The model under review builds one solid part; all positions refer to its coordinate system, in mm. A direction names the side the tool comes from. Coordinates: 2 decimals unless noted, no trailing zeros. Write each loop counter-clockwise with the first axis right and the second up, starting at its lowest first coordinate (ties: lowest second). Pieces come first, ordered by that corner, then holes. Notation, with made-up numbers: (74.5, 53) - (117.5, 53) arc R11 ccw to (117.5, 69) - close; hole circle Ø6 at (37.25, -14.75). An arc over 180 degrees is marked (long way). Put each result on its own line as item: value. Start each with the question number.
Item 1: Mouldability with a two-part tool opening along X and no side actions: class faces 1 (the face through (7, 0, 20)), 2 (the face through (-28, -21, 15)), 3 (the face through (18.34, 1.05, 17.46)) as pulls with the +X half, pulls with the -X half, needs draft (parallel to the pull), parting line crosses it, or undercut.
Item 2: Machinability: for faces 4 (the face through (-11.66, 1.05, 17.46)), 5 (the face through (8, 0, 12)), which of the approach directions +Z, -Z, +X, -X, +Y, -Y give a long, thin tool a straight path to every point of the face, cutting with its end or side? Answer none if there is none.
Item 3: Consider section B-B on z = 16.5. Give the boundary of the cut face in (x, y), then the cut area to 3 significant figures.
Item 4: Consider section A-A on x = 0. Give the boundary of the cut face in (y, z), then the cut area to 3 significant figures.
Item 5: To check wall thickness, follow L1, parallel to Y at x = 25, z = 15; L2, parallel to Y at x = 15, z = 18.8; L3, parallel to X at y = 14, z = 17.75. State the ranges of each line that lie inside material, in increasing order. Write a range as [from, to].
Item 6: For pin 1 (3 mm diameter, centred on x = 9, z = 16.5, fed in from -Y); pin 2 (8.5 mm diameter, centred on x = 15, y = 0, fed in from -Z); pin 3 (6 mm diameter, centred on x = -18, z = 16.5, fed in from -Y), all flat-tipped, find the tip position at first contact; note any pin that passes through.
```python
from build123d import *

# Parameters (mm, degrees)
CYLINDER001_R        = 3.5
CYLINDER001_DEPTH    = 10
CYLINDER002_R        = 7
CYLINDER002_DEPTH    = 5
CYLINDER003_R        = 3.5
CYLINDER003_DEPTH    = 10
CYLINDER004_R        = 7
CYLINDER004_DEPTH    = 5
CYLINDER005_R        = 2.6
CYLINDER005_DEPTH    = 10
CYLINDER006_R        = 2.6
CYLINDER006_DEPTH    = 10
CYLINDER_R           = 3
CYLINDER_DEPTH       = 10
CYLINDER001027_R     = 35
CYLINDER001027_DEPTH = 10
CHAMFER004_SIZE      = 1


with BuildPart() as cylinder001:
    # cylinder001 → cylinder001 (new body)
    with BuildSketch(Plane(origin=(15, 0, 0), x_dir=(1, 0, 0), z_dir=(0, 0, 1))):
        Circle(CYLINDER001_R)
    extrude(amount=CYLINDER001_DEPTH)


with BuildPart() as cylinder002:
    # cylinder002 → cylinder002 (new body)
    with BuildSketch(Plane(origin=(15, 0, 0), x_dir=(1, 0, 0), z_dir=(0, 0, 1))):
        Circle(CYLINDER002_R)
    extrude(amount=CYLINDER002_DEPTH)


with BuildPart() as cylinder003:
    # cylinder003 → cylinder003 (new body)
    with BuildSketch(Plane(origin=(-15, 0, 0), x_dir=(1, 0, 0), z_dir=(0, 0, 1))):
        Circle(CYLINDER003_R)
    extrude(amount=CYLINDER003_DEPTH)


with BuildPart() as cylinder004:
    # cylinder004 → cylinder004 (new body)
    with BuildSketch(Plane(origin=(-15, 0, 0), x_dir=(1, 0, 0), z_dir=(0, 0, 1))):
        Circle(CYLINDER004_R)
    extrude(amount=CYLINDER004_DEPTH)


with BuildPart() as cylinder005:
    # cylinder005 → cylinder005 (new body)
    with BuildSketch(Plane(origin=(-25, 0, 0), x_dir=(1, 0, 0), z_dir=(0, 0, 1))):
        Circle(CYLINDER005_R)
    extrude(amount=CYLINDER005_DEPTH)


with BuildPart() as cylinder006:
    # cylinder006 → cylinder006 (new body)
    with BuildSketch(Plane(origin=(25, 0, 0), x_dir=(1, 0, 0), z_dir=(0, 0, 1))):
        Circle(CYLINDER006_R)
    extrude(amount=CYLINDER006_DEPTH)


with BuildPart() as union:
    # cylinder → cylinder (new body)
    with BuildSketch(Plane.XY):
        Circle(CYLINDER_R)
    extrude(amount=CYLINDER_DEPTH)

    # union: union cylinder001, cylinder002, cylinder003, cylinder004, cylinder005, cylinder006
    add(cylinder001.part)
    add(cylinder002.part)
    add(cylinder003.part)
    add(cylinder004.part)
    add(cylinder005.part)
    add(cylinder006.part)


with BuildPart() as obj1:
    # Cylinder001027 → Cylinder001027 (new body)
    with BuildSketch(Plane.XY):
        Circle(CYLINDER001027_R)
    extrude(amount=CYLINDER001027_DEPTH)

    # Cut004: cut union
    add(union.part, mode=Mode.SUBTRACT)


with BuildPart() as obj1_1:
    # Cut004 placement: moved
    add(obj1.part.moved(Location((0, 0, 10))))

    # Chamfer004
    chamfer004_edges = [obj1_1.edges().sort_by_distance(p)[0] for p in [
        (-35, 0, 20),
        (-35, 0, 10),
    ]]
    chamfer(chamfer004_edges, length=CHAMFER004_SIZE)


solid = obj1_1.part
```
Report:
1. face 1: needs draft
1. face 2: parting line crosses it
1. face 3: undercut
2. face 4: +Z, -Z
2. face 5: -Z
3. outline: circle Ø70 at (0, 0); hole circle Ø5.2 at (-25, 0); hole circle Ø7 at (-15, 0); hole circle Ø6 at (0, 0); hole circle Ø7 at (15, 0); hole circle Ø5.2 at (25, 0)
3. area: 3,700 mm²
4. outline: (-35, 11) - (-34, 10) - (-3, 10) - (-3, 20) - (-34, 20) - (-35, 19) - close; (3, 10) - (34, 10) - (35, 11) - (35, 19) - (34, 20) - (3, 20) - close
4. area: 638 mm²
5. L1: [-24.49, -2.6], [2.6, 24.49]
5. L2: [-31.62, -3.5], [3.5, 31.62]
5. L3: [-32.08, 32.08]
6. pin 1: y = -34.19
6. pin 2: z = 15
6. pin 3: y = -31.62
